Geometry: final body of the model. Coordinates: model frame, mm. A direction names the side the tool comes from. Give positions to 0.01 mm unless a question says otherwise; leave off trailing zeros. Write each loop counter-clockwise with the first axis right and the second up, starting at its lowest first coordinate (ties: lowest second). Pieces come first, ordered by that corner, then holes.
Q1. Line query: line 1 (X direction, y = 10.5, z = 0.55); line 2 (Y direction, x = 25.5, z = 0.55); line 3 (Y direction, x = 30, z = 2.15). Output: solid intervals per line, ascending.
Q2. Section B-B (x = 37). Return the cut outline in (y, z), plus the area to 3 significant figures.
Q3. Section D-D (z = 1.9). Return the cut outline in (x, y).
Q4. Mould query, pull axis Y, two halves, no side actions, for faces 1 (the flat face through (55, 1.2, 3)), 2 (the flat face through (45.57, 3, 1)), 3 (the flat face through (50, 7, 6)). Classes: +Y half, -Y half, draft (parallel to the pull), parting line (faces both ways), or undercut.
Q5. Pin query (flat end, axial travel): pin 1 Ø1 at (y, z) = (10.5, 5.5) entering from -X; pin 2 Ø1.3 at (x, z) = (55, 3) entering from +Y; pin 3 Ø1.5 at (x, y) = (17, 2.5) entering from +Z; pin 4 Ø2 at (x, y) = (11.5, 9.5) entering from +Z. Return the tip coordinate at first contact, or that it passes through.
Q6. Reachability of faces 4 (the flat face through (1, 7, 4)), 5 (the flat face through (10.1, 2.5, 0.5)), 6 (the flat face through (35, 13, 3.25)) from +Z, -Z, +X, -X, +Y, -Y: full face, straight path, thin tool, end or side. Return the list, or none.
Q7. Section C-C (y = 8). Return the cut outline in (x, z).
Q8. Section A-A (y = 3.25). Return the cut outline in (x, z).
from build123d import *
from OCP.BRepFilletAPI import BRepFilletAPI_MakeChamfer

# Parameters (mm, degrees)
ESQUISSE1_W             = 20.32
ESQUISSE1_H             = 13.2
BOSS_EXTRU_1_DEPTH      = 6
ESQUISSE2_W             = 18.32
ESQUISSE2_H             = 11.2
ENL_V_MAT_EXTRU_1_DEPTH = 5
ESQUISSE3_W             = 5
ESQUISSE3_H             = 1
ENL_V_MAT_EXTRU_2_DEPTH = 5
ESQUISSE4_W             = 15.32
ESQUISSE4_H             = 8.2
ENL_V_MAT_EXTRU_3_DEPTH = 25.741511676
ESQUISSE6_W             = 1
ESQUISSE6_H             = 11.2
ENL_V_MAT_EXTRU_4_DEPTH = 4.75
ESQUISSE7_W             = 30
ESQUISSE7_H             = 13.2
BOSS_EXTRU_2_DEPTH      = 1.25
ESQUISSE8_W             = 1.25
ESQUISSE8_H             = 13.2
BOSS_EXTRU_3_DEPTH      = 4.75
ESQUISSE9_W             = 6
ESQUISSE9_H             = 1.25
BOSS_EXTRU_4_DEPTH      = 6
CHANFREIN1_SIZE         = 2
CHANFREIN1_SIZE_2       = 3.464101615
ESQUISSE10_W            = 28.75
ESQUISSE10_H            = 1
BOSS_EXTRU_5_DEPTH      = 2
CHANFREIN2_SIZE         = 2
CHANFREIN2_SIZE2        = 3.464101615
ESQUISSE11_W            = 21
ESQUISSE11_H            = 1.433492253
ENL_V_MAT_EXTRU_5_DEPTH = 2


with BuildPart() as part:
    # Esquisse1 → Boss.-Extru.1 (new body)
    with BuildSketch(Plane.XY):
        with Locations((10.16, 6.6)):
            Rectangle(ESQUISSE1_W, ESQUISSE1_H)
    extrude(amount=BOSS_EXTRU_1_DEPTH)

    # Esquisse2 → Enlèv. mat.-Extru.1 (cut)
    with BuildSketch(Plane.XY.offset(6)):
        with Locations((10.16, 6.6)):
            Rectangle(ESQUISSE2_W, ESQUISSE2_H)
    extrude(amount=-ENL_V_MAT_EXTRU_1_DEPTH, mode=Mode.SUBTRACT)

    # Esquisse3 → Enlèv. mat.-Extru.2 (cut)
    with BuildSketch(Plane.XY.offset(6)):
        with Locations((3.5, 12.7)):
            Rectangle(ESQUISSE3_W, ESQUISSE3_H)
    extrude(amount=-ENL_V_MAT_EXTRU_2_DEPTH, mode=Mode.SUBTRACT)

    # Esquisse4 → Enlèv. mat.-Extru.3 (cut, through all)
    with BuildSketch(Plane.XY.offset(1)):
        with Locations((10.16, 6.6)):
            Rectangle(ESQUISSE4_W, ESQUISSE4_H)
    extrude(amount=-ENL_V_MAT_EXTRU_3_DEPTH, mode=Mode.SUBTRACT)

    # Esquisse6 → Enlèv. mat.-Extru.4 (cut)
    with BuildSketch(Plane.XY.offset(6)):
        with Locations((19.82, 6.6)):
            Rectangle(ESQUISSE6_W, ESQUISSE6_H)
    extrude(amount=-ENL_V_MAT_EXTRU_4_DEPTH, mode=Mode.SUBTRACT)

    # Esquisse7 → Boss.-Extru.2 (add)
    with BuildSketch(Plane(origin=(0, 0, 0), x_dir=(-1, 0, 0), z_dir=(0, 0, -1))):
        with Locations((-35.32, 6.6)):
            Rectangle(ESQUISSE7_W, ESQUISSE7_H)
    extrude(amount=-BOSS_EXTRU_2_DEPTH)

    # Esquisse8 → Boss.-Extru.3 (add)
    with BuildSketch(Plane.XY.offset(1.25)):
        with Locations((49.695, 6.6)):
            Rectangle(ESQUISSE8_W, ESQUISSE8_H)
    extrude(amount=BOSS_EXTRU_3_DEPTH)

    # Esquisse9 → Boss.-Extru.4 (add)
    with BuildSketch(Plane(origin=(50.32, 0, 0), x_dir=(0, 0, -1), z_dir=(1, 0, 0))):
        with Locations((-3, 11.375)):
            Rectangle(ESQUISSE9_W, ESQUISSE9_H)
        with Locations((-3, 1.825)):
            Rectangle(ESQUISSE9_W, ESQUISSE9_H)
    extrude(amount=BOSS_EXTRU_4_DEPTH)

    # Chanfrein1
    # the kernel refuses this chamfer: 3.464101615, 2 mm, written as the material it adds along each edge
    with BuildSketch(Plane(origin=(50.32, 12, 6), x_dir=(-0.057893862402669756, 0.9983227437537926, 0), z_dir=(0, 0, -1))) as chanfrein1_piece_1_section:
        Polygon((CHANFREIN1_SIZE * 0.998322743754, CHANFREIN1_SIZE * 0.0578938624027), (-CHANFREIN1_SIZE_2 * 0.057893862405, CHANFREIN1_SIZE_2 * 0.998322743793), (0, 0), align=None)
    chanfrein1_piece_1 = extrude(amount=6, mode=Mode.PRIVATE)
    chanfrein1_piece_1 = split(chanfrein1_piece_1, bisect_by=Plane(origin=(51.640549775, 13.2, 3), z_dir=(0, -1, 0)), keep=Keep.TOP, mode=Mode.PRIVATE)
    add(chanfrein1_piece_1)
    with BuildSketch(Plane(origin=(50.32, 1.2, 0), x_dir=(-0.05789386240266974, -0.9983227437537926, 0), z_dir=(0, 0, 1))) as chanfrein1_piece_2_section:
        Polygon((CHANFREIN1_SIZE * 0.998322743754, CHANFREIN1_SIZE * 0.0578938624027), (-CHANFREIN1_SIZE_2 * 0.057893862405, CHANFREIN1_SIZE_2 * 0.998322743793), (0, 0), align=None)
    chanfrein1_piece_2 = extrude(amount=6, mode=Mode.PRIVATE)
    chanfrein1_piece_2 = split(chanfrein1_piece_2, bisect_by=Plane(origin=(51.640549775, 0, 3), z_dir=(0, 1, 0)), keep=Keep.TOP, mode=Mode.PRIVATE)
    add(chanfrein1_piece_2)

    # Esquisse10 → Boss.-Extru.5 (add)
    with BuildSketch(Plane.XY.offset(1.25)):
        with Locations((34.695, 12.7)):
            Rectangle(ESQUISSE10_W, ESQUISSE10_H)
        with Locations((34.695, 0.5)):
            Rectangle(ESQUISSE10_W, ESQUISSE10_H)
    extrude(amount=BOSS_EXTRU_5_DEPTH)

    # Chanfrein2: one chamfer whose edges measure the first distance from different faces: ONE call of the kernel's chamfer builder (chamfer() names one face for all edges)
    chanfrein2_edges_1 = [part.edges().sort_by_distance(p)[0] for p in [
        (20.32, 12.7, 3.25),
    ]]
    chanfrein2_side_1 = [part.faces().sort_by_distance(p)[0] for p in [
        (20.32, 12.7, 4.625),
    ]]
    chanfrein2_edges_2 = [part.edges().sort_by_distance(p)[0] for p in [
        (49.07, 12.7, 3.25),
        (49.07, 0.5, 3.25),
    ]]
    chanfrein2_side_2 = [part.faces().sort_by_distance(p)[0] for p in [
        (49.07, 6.6, 3.718696763),
    ]]
    chanfrein2_edges_3 = [part.edges().sort_by_distance(p)[0] for p in [
        (20.32, 0.5, 3.25),
    ]]
    chanfrein2_side_3 = [part.faces().sort_by_distance(p)[0] for p in [
        (20.32, 0.5, 4.625),
    ]]
    chanfrein2 = BRepFilletAPI_MakeChamfer(part.part.solid().wrapped)
    for e in chanfrein2_edges_1:
        chanfrein2.Add(CHANFREIN2_SIZE, CHANFREIN2_SIZE2, e.wrapped, chanfrein2_side_1[0].wrapped)  # the first distance lies on this face
    for e in chanfrein2_edges_2:
        chanfrein2.Add(CHANFREIN2_SIZE, CHANFREIN2_SIZE2, e.wrapped, chanfrein2_side_2[0].wrapped)  # the first distance lies on this face
    for e in chanfrein2_edges_3:
        chanfrein2.Add(CHANFREIN2_SIZE, CHANFREIN2_SIZE2, e.wrapped, chanfrein2_side_3[0].wrapped)  # the first distance lies on this face
    add(Compound.cast(chanfrein2.Shape()), mode=Mode.REPLACE)

    # Esquisse11 → Enlèv. mat.-Extru.5 (cut)
    with BuildSketch(Plane.XY.offset(1.25)):
        with Locations((35.07, 9.983253874)):
            Rectangle(ESQUISSE11_W, ESQUISSE11_H)
        with Locations((35.07, 6.683253873)):
            Rectangle(ESQUISSE11_W, ESQUISSE11_H)
        with Locations((35.07, 3.383253874)):
            Rectangle(ESQUISSE11_W, ESQUISSE11_H)
    extrude(amount=-ENL_V_MAT_EXTRU_5_DEPTH, mode=Mode.SUBTRACT)


solid = part.part
Computed:
1. line 1: x = 0 to 2.5, 17.82 to 24.57, 45.57 to 50.32
1. line 2: y = 0 to 2.67, 4.1 to 5.97, 7.4 to 9.27, 10.7 to 13.2
1. line 3: y = 0 to 1, 12.2 to 13.2
2. outline: (0, 0) - (2.67, 0) - (2.67, 1.25) - (1, 1.25) - (1, 3.25) - (0, 3.25) - close; (4.1, 0) - (5.97, 0) - (5.97, 1.25) - (4.1, 1.25) - close; (7.4, 0) - (9.27, 0) - (9.27, 1.25) - (7.4, 1.25) - close; (10.7, 0) - (13.2, 0) - (13.2, 3.25) - (12.2, 3.25) - (12.2, 1.25) - (10.7, 1.25) - close
2. area: 15.1 mm2
3. outline: (0, 0) - (51.71, 0) - (53.78, 1.2) - (56.32, 1.2) - (56.32, 2.45) - (50.32, 2.45) - (50.32, 10.75) - (56.32, 10.75) - (56.32, 12) - (53.78, 12) - (51.71, 13.2) - (6, 13.2) - (6, 12.2) - (49.07, 12.2) - (49.07, 1) - (1, 1) - (1, 13.2) - (0, 13.2) - close
4. face 1: -Y half
4. face 2: undercut
4. face 3: draft
5. pin 1: stops at x = 0
5. pin 2: stops at y = 12
5. pin 3: stops at z = 1
5. pin 4: passes through
6. face 4: +Z, +Y
6. face 5: +Z, -Z
6. face 6: +Z, +Y, -Y
7. outline: (0, 0) - (2.5, 0) - (2.5, 1) - (1, 1) - (1, 6) - (0, 6) - close; (17.82, 0) - (50.32, 0) - (50.32, 6) - (49.07, 6) - (49.07, 1.25) - (19.32, 1.25) - (19.32, 1) - (17.82, 1) - close
8. outline: (0, 0) - (2.5, 0) - (2.5, 1) - (1, 1) - (1, 6) - (0, 6) - close; (17.82, 0) - (24.57, 0) - (24.57, 1.25) - (19.32, 1.25) - (19.32, 1) - (17.82, 1) - close; (45.57, 0) - (50.32, 0) - (50.32, 6) - (49.07, 6) - (49.07, 1.25) - (45.57, 1.25) - close
